```python
from build123d import *

# Parameters (mm, degrees)
BOSS_EXTRUDE1_DEPTH = 5
SKETCH2_R           = 2.25
CUT_EXTRUDE1_DEPTH  = 8.141428429


with BuildPart() as part:
    # Sketch1 → Boss-Extrude1 (new, symmetric)
    with BuildSketch(Plane.XY):
        with BuildLine():
            Line((-5, 0), (5, 0))
            Line((5, 0), (5, -1))
            ThreePointArc((5, -1), (0, -0.631439341), (-5, -1))
            Line((-5, -1), (-5, 0))
        make_face()
    extrude(amount=BOSS_EXTRUDE1_DEPTH, both=True)

    # Sketch2 → Cut-Extrude1 (cut, through all)
    with BuildSketch(Plane(origin=(0, 0, 0), x_dir=(1, 0, 0), z_dir=(0, 1, 0))):
        with Locations(Location((0, 0, 0), (0, 0, 180))):
            Circle(SKETCH2_R)
    extrude(amount=-CUT_EXTRUDE1_DEPTH, mode=Mode.SUBTRACT)


solid = part.part
```
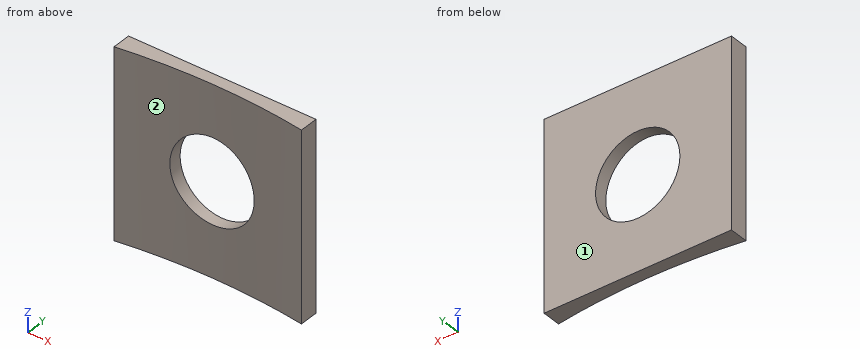
Source: CAD feature listing. Evaluate the final solid. Frame: model axes, mm. Face numbers are marked on the shaded views. Coordinates: 2 decimals unless noted, no trailing zeros. Write each loop counter-clockwise with the first axis right and the second up, starting at its lowest first coordinate (ties: lowest second). Pieces come first, ordered by that corner, then holes. Notation, with made-up numbers: (15, 83.5) - (42, 83.5) arc R28 ccw to (42, 116.5) - close; hole circle Ø8 at (-9.75, -14). An arc over 180 degrees is marked (long way). Answer as a JSON object with one key per item and string values.
Q1. Section query A-A, the plane x = 0. Output: boundary loops of the cut face in (y, z).
Ans:
{"outline": "(-0.63, -5) - (0, -5) - (0, -2.25) - (-0.63, -2.25) - close; (-0.63, 2.25) - (0, 2.25) - (0, 5) - (-0.63, 5) - close"}
Q2. Section query B-B, the plane z = 0. Output: boundary loops of the cut face in (x, y).
Ans:
{"outline": "(-5, -1) arc R34.1 cw to (-2.25, -0.71) - (-2.25, 0) - (-5, 0) - close; (2.25, -0.71) arc R34.1 cw to (5, -1) - (5, 0) - (2.25, 0) - close"}
Q3. Section query D-D, the plane z = -3.75. Output: boundary loops of the cut face in (x, y).
Ans:
{"outline": "(-5, -1) arc R34.1 cw to (5, -1) - (5, 0) - (-5, 0) - close"}
Q4. Material intervals for line 1 (Z direction, x = 0, y = -0.15); line 2 (X direction, y = -0.6, z = -1), sorted ascending. Write a range as [from, to].
Ans:
{"line 1": "z = [-5, -2.25], [2.25, 5]", "line 2": "x = [-5, -2.02], [2.02, 5]"}
Q5. First-contact query: pin 1 Ø5 at (x, z) = (1, 0.5) entering from -Y. Flat tip, straight axial feed; report the tip coordinate or a pass-through.
Ans:
{"pin 1": "stops at y = -0.81"}
Q6. Draft query along X for the marked faces 1 and 2. Return one class per face: released by +X, released by -X, zero draft, split by the parting line, or undercut.
Ans:
{"face 1": "zero draft", "face 2": "undercut"}
Q7. Section query C-C, the plane y = -0.2. Output: boundary loops of the cut face in (x, z).
Ans:
{"outline": "(-5, -5) - (5, -5) - (5, 5) - (-5, 5) - close; hole circle Ø4.5 at (0, 0)"}
